from build123d import *


with BuildPart() as f2:
    # F1 (on Front) → F2 (revolve)
    with BuildSketch(Plane.XZ):
        with BuildLine():
            Line((0, 78.8675134595), (0, -21.1324865405))
            ThreePointArc((0, -21.1324865405), (50, 28.8675134595), (0, 78.8675134595))
        make_face()
    revolve(axis=Axis((0, 0, 42.5087921321), (0, 0, 1)))


with BuildPart() as f4:
    # F3 (on Front) → F4 (revolve)
    with BuildSketch(Plane.XZ):
        with BuildLine():
            Line((18.3012701892, 10.5662432703), (-68.3012701892, -39.4337567297))
            ThreePointArc((-68.3012701892, -39.4337567297), (0, -57.735026919), (18.3012701892, 10.5662432703))
        make_face()
    revolve(axis=Axis((-48.7220736529, 0, -28.129702339), (-0.8660254038, 0, -0.5)))


with BuildPart() as f6:
    # F5 (on Front) → F6 (revolve)
    with BuildSketch(Plane.XZ):
        with BuildLine():
            Line((68.3012701892, -39.4337567297), (-18.3012701892, 10.5662432703))
            ThreePointArc((-18.3012701892, 10.5662432703), (0, -57.735026919), (68.3012701892, -39.4337567297))
        make_face()
    revolve(axis=Axis((48.6017106384, 0, -28.0602107202), (0.8660254038, 0, -0.5)))


with BuildPart() as f10:
    # F9 (on Top) → F10 (revolve)
    with BuildSketch(Plane.XY):
        with BuildLine():
            Line((0, -93.3012701892), (0, 6.6987298108))
            ThreePointArc((0, 6.6987298108), (-50, -43.3012701892), (0, -93.3012701892))
        make_face()
    revolve(axis=Axis((0, -54.9783110619, 0), (0, -1, 0)))


with BuildPart() as f2_1:
    add(f2.part)

    # F11: intersect F4, F6, F10
    add(f4.part, mode=Mode.INTERSECT)
    add(f6.part, mode=Mode.INTERSECT)
    add(f10.part, mode=Mode.INTERSECT)


solid = f2_1.part
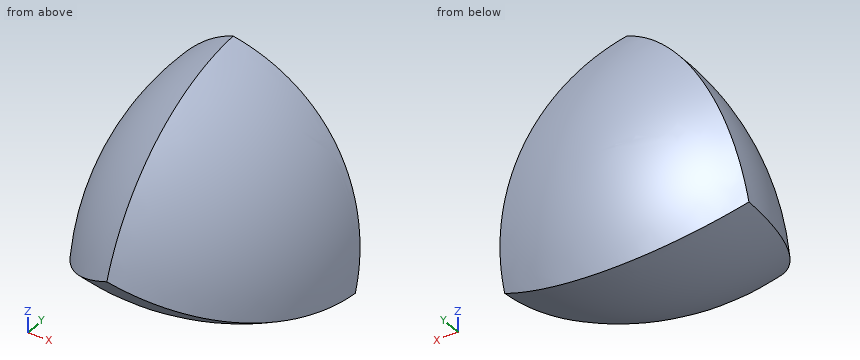
Design review of the part built by this model. Coordinates are the model's own, in mm. Coordinates: 2 decimals unless noted, no trailing zeros. Order: outer loops, then holes, each group sorted by start corner. A loop starts at its lowest first (then second) coordinate and runs counter-clockwise, first axis right, second up. Notation, with made-up numbers: M 11,78 L 51,78 A8 ccw 51,88 Z; hole C 26,81.5 d9. An arc over 180 degrees is marked long. Use a Markdown table: item, result.
(1) Add section B-B (x = 21). Give the boundary of the cut face in (y, z), then the cut area to 3 significant figures.
Worked answers:
| item | result |
|---|---|
| outline | M -19.46,-12.12 A45.38 ccw -1.03,-16.5 A45.38 ccw 1.79,5.08 A19.6 ccw Z |
| area | 341 mm2 |
(2) Add section A-A (y = -23.5). Give the boundary of the cut face in (x, z), then the cut area to 3 significant figures.
Worked answers:
| item | result |
|---|---|
| outline | M -19,-10.97 A44.13 ccw 19,-10.97 A44.13 ccw 0,21.94 A44.13 ccw Z |
| area | 955 mm2 |
(3) Add section C-C (z = -4). Give the boundary of the cut face in (x, y), then the cut area to 3 significant figures.
Worked answers:
| item | result |
|---|---|
| outline | M -23.9,0.44 A48.9 ccw -6.93,-37.04 A37.68 ccw 6.93,-37.04 A48.9 ccw 23.9,0.44 A49.84 ccw Z |
| area | 1,610 mm2 |
(4) Wall thickness on probe 1 along Z at (x, y) = (-9.5, 2); probe 2 along X at (y, z) = (-26, -1); probe 3 along Y at (x, z) = (4.5, 21): over which ranges is each line inside the solid? List them lowest first.
Worked answers:
| item | result |
|---|---|
| probe 1 | z = -18.91 to 18.91 |
| probe 2 | x = -15.54 to 15.54 |
| probe 3 | y = -19.34 to 1.85 |
(5) For P1, Ø2, axis at y = -6.5, z = 19, coming from the -X side; P2, Ø8, axis at y = -20.5, z = 6.5, coming from the -X side; P3, Ø3, axis at x = -11, y = -25.5, coming from the +Z side, all flat-tipped, find the tip position at first contact; note any pin that passes through.
Worked answers:
| item | result |
|---|---|
| P1 | stops at x = -12.51 |
| P2 | stops at x = -18.13 |
| P3 | stops at z = 11.72 |
(6) Add section D-D (y = 4). Give the boundary of the cut face in (x, z).
Worked answers:
| item | result |
|---|---|
| outline | C 0,0 d32.41 |
